Part print with two shaded views. Sizes in mm from the minimum x, y, z corner. Give positions to 0.01 mm unless a question says otherwise; leave off trailing zeros. Write each loop counter-clockwise with the first axis right and the second up, starting at its lowest first coordinate (ties: lowest second). Pieces come first, ordered by that corner, then holes.
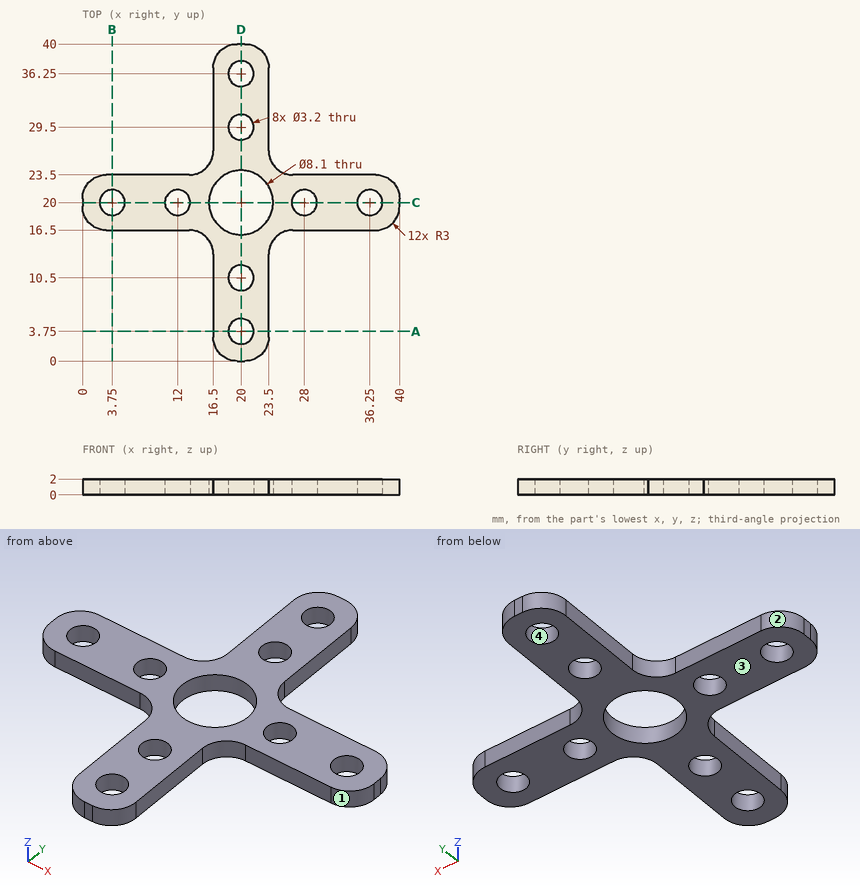
(1) Probe line 1 (Y direction, x = 20, z = 0.95); line 2 (Y direction, x = 3.75, z = 0.55); line 3 (Y direction, x = 8.5, z = 0.5). List the from-to ranges inside material, lowest first.
(2) Saw through at C-C, the plane y = 20. List the corners of the cut face in (x, z).
(3) Mould opens along Y. For the marked faces 1, 2, 3 and 4 say: +Y half, -Y half, draft (parallel to the pull), parting line (faces both ways), or undercut.
(4) Saw through at A-A, the plane y = 3.75. List the corners of the cut face in (x, z).
(5) Saw through at D-D, the plane x = 20. List the corners of the cut face in (y, z), plus the area to 3 significant figures.
(6) Drop flat-ended pins along their axis: pin 1 (3 mm diameter, centred on x = 28, y = 20, fed in from -Z); pin 2 (5 mm diameter, centred on x = 20, y = 36.25, fed in from -Z); pin 3 (1 mm diameter, centred on x = 31.5, z = 1.5, fed in from +Y); pin 4 (0.6 mm diameter, centred on y = 29, z = 1, fed in from +X). Give the stop position or say it passes through.
Computed values:
1. line 1: y = 0 to 2.15, 5.35 to 8.9, 12.1 to 15.95, 24.05 to 27.9, 31.1 to 34.65, 37.85 to 40
1. line 2: y = 16.5 to 18.4, 21.6 to 23.5
1. line 3: y = 16.5 to 23.5
2. outline: (0, 0) - (2.15, 0) - (2.15, 2) - (0, 2) - close; (5.35, 0) - (10.4, 0) - (10.4, 2) - (5.35, 2) - close; (13.6, 0) - (15.95, 0) - (15.95, 2) - (13.6, 2) - close; (24.05, 0) - (26.4, 0) - (26.4, 2) - (24.05, 2) - close; (29.6, 0) - (34.65, 0) - (34.65, 2) - (29.6, 2) - close; (37.85, 0) - (40, 0) - (40, 2) - (37.85, 2) - close
3. face 1: -Y half
3. face 2: +Y half
3. face 3: draft
3. face 4: undercut
4. outline: (16.5, 0) - (18.4, 0) - (18.4, 2) - (16.5, 2) - close; (21.6, 0) - (23.5, 0) - (23.5, 2) - (21.6, 2) - close
5. outline: (0, 0) - (2.15, 0) - (2.15, 2) - (0, 2) - close; (5.35, 0) - (8.9, 0) - (8.9, 2) - (5.35, 2) - close; (12.1, 0) - (15.95, 0) - (15.95, 2) - (12.1, 2) - close; (24.05, 0) - (27.9, 0) - (27.9, 2) - (24.05, 2) - close; (31.1, 0) - (34.65, 0) - (34.65, 2) - (31.1, 2) - close; (37.85, 0) - (40, 0) - (40, 2) - (37.85, 2) - close
5. area: 38.2 mm2
6. pin 1: passes through
6. pin 2: stops at z = 0
6. pin 3: stops at y = 23.5
6. pin 4: stops at x = 23.5
